```python
from build123d import *

# Parameters (mm, degrees)
F0_W     = 280
F0_H     = 40
F1_DEPTH = 160
F2_R     = 5
F3_R     = 7.5
F4_DEPTH = 50
F5_DEPTH = 100
F7_DEPTH = 81751


with BuildPart() as f1:
    # F0 (on Right) → F1 (new body, symmetric)
    with BuildSketch(Plane.YZ):
        with Locations((10.9808796245, -66.3028520482)):
            Rectangle(F0_W, F0_H)
    extrude(amount=F1_DEPTH, both=True)

    # F2
    f2_edges = [f1.edges().sort_by_distance(p)[0] for p in [
        (160, -129.01912, -66.302852),
        (-160, -129.01912, -66.302852),
        (160, 150.98088, -66.302852),
        (-160, 150.98088, -66.302852),
    ]]
    fillet(f2_edges, radius=F2_R)

    # F3 (on face) → F4 (cut)
    with BuildSketch(Plane(origin=(0, 0, -86.3028520482), x_dir=(1, 0, 0), z_dir=(0, 0, -1))):
        with Locations((130, -80.9808796245)):
            Circle(F3_R)
        with Locations((130, 59.0191203755)):
            Circle(F3_R)
        with Locations((-130, -80.9808796245)):
            Circle(F3_R)
        with Locations((-130, 59.0191203755)):
            Circle(F3_R)
    extrude(amount=-F4_DEPTH, mode=Mode.SUBTRACT)

    # F0 (on Right) → F5 (join, symmetric)
    with BuildSketch(Plane.YZ):
        Polygon((20.9808796245, 157.6971479518), (-129.0191203755, 7.6971479518), (-129.0191203755, -46.3028520482), (150.9808796245, -46.3028520482), (150.9808796245, 77.6971479518), (70.9808796245, 157.6971479518), align=None)
    extrude(amount=F5_DEPTH, both=True)

    # F6 (on face) → F7 (cut)
    with BuildSketch(Plane(origin=(0, -68.3581341637, 68.3581341637), x_dir=(1, 0, 0), z_dir=(0, -0.7071067812, 0.7071067812))):
        with BuildLine():
            Line((0, -48.4145147354), (0, 101.5854852646))
            ThreePointArc((0, 101.5854852646), (-75, 26.5854852646), (0, -48.4145147354))
        make_face()
        with BuildLine():
            ThreePointArc((75, 26.5854852646), (53.033008589, 79.6184938536), (0, 101.5854852646))
            Line((0, 101.5854852646), (0, -48.4145147354))
            ThreePointArc((0, -48.4145147354), (53.033008589, -26.4475233244), (75, 26.5854852646))
        make_face()
    extrude(amount=-F7_DEPTH, mode=Mode.SUBTRACT)


solid = f1.part
```
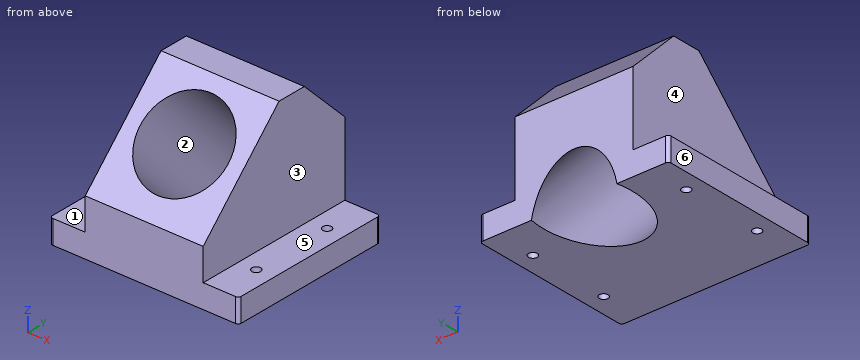
Design review of the part built by this model. Coordinates are the model's own, in mm. Face numbers are marked on the shaded views. A direction names the side the tool comes from. Give positions to 0.01 mm unless a question says otherwise; leave off trailing zeros. Order: outer loops, then holes, each group sorted by start corner. A loop starts at its lowest first (then second) coordinate and runs counter-clockwise, first axis right, second up. Notation, with made-up numbers: M 41.5,-32 L 87.5,-32 A11 cw 87.5,-18 Z; hole C 9.25,29 d4. An arc over 180 degrees is marked long. One line per question, with ' | ' between items. Start each with the question number.
Q1. The part is to be moulded in two halves that separate along Z. For the marked faces 1, 2 and 3, say which applies: +Z half, -Z half, draft (parallel to the pull), parting line (faces both ways), or undercut.
Q2. We need section C-C (x = -87). Write out the cut boundary in (y, z), plus the area to 3 significant figures.
Q3. Machinability: for the marked faces 4, 5 and 6, which of the approach directions +Z, -Z, +X, -X, +Y, -Y give a long, thin tool a straight path to every point of the face, cutting with its end or side? Answer none if there is none.
Q4. We need section B-B (x = 66). Write out the cut boundary in (y, z), plus the area to 3 significant figures.
Q5. For pin 1 Ø1 at (x, z) = (-1, 108.5) entering from +Y; pin 2 Ø6 at (y, z) = (80.5, 20) entering from +X; pin 3 Ø8 at (y, z) = (104.5, 129.5) entering from -X; pin 4 Ø24 at (x, y) = (130, -59.02) entering from -Z, all flat-tipped, find the tip position at first contact; note any pin that passes through.
Q6. We need section A-A (x = -130). Write out the cut boundary in (y, z), plus the area to 3 significant figures.
Q7. For L1, parallel to Y at x = 130, z = -60.5; L2, parallel to X at y = 109.5, z = -69; L3, parallel to X at y = 34, z = 70, list the stretches that pass through material, from the lowest coordinate up. Write a range as [from, to].
Returned:
1) face 1: +Z half | face 2: undercut | face 3: draft
2) outline: M -129.02,-86.3 L 150.98,-86.3 L 150.98,77.7 L 70.98,157.7 L 20.98,157.7 L -129.02,7.7 Z | area: 53,900 mm2
3) face 4: +Z, -X, +Y, -Y | face 5: +Z, +X, +Y, -Y | face 6: +Z, -Z, -X, +Y, -Y
4) outline: M -129.02,-86.3 L 73.52,-86.3 L -74.75,61.97 L -129.02,7.7 Z; M -24.37,112.35 L 150.98,-63 L 150.98,77.7 L 70.98,157.7 L 20.98,157.7 Z | area: 36,700 mm2
5) pin 1: y = 120.68 | pin 2: x = 100 | pin 3: x = -100 | pin 4: z = -86.3
6) outline: M -129.02,-86.3 L -66.52,-86.3 L -66.52,-46.3 L -129.02,-46.3 Z; M -51.52,-86.3 L 73.48,-86.3 L 73.48,-46.3 L -51.52,-46.3 Z; M 88.48,-86.3 L 150.98,-86.3 L 150.98,-46.3 L 88.48,-46.3 Z | area: 10,000 mm2
7) L1: [-129.02, -66.52], [-51.52, 73.48], [88.48, 150.98] | L2: [-160, -74.97], [74.97, 160] | L3: [-100, -58.48], [58.48, 100]
